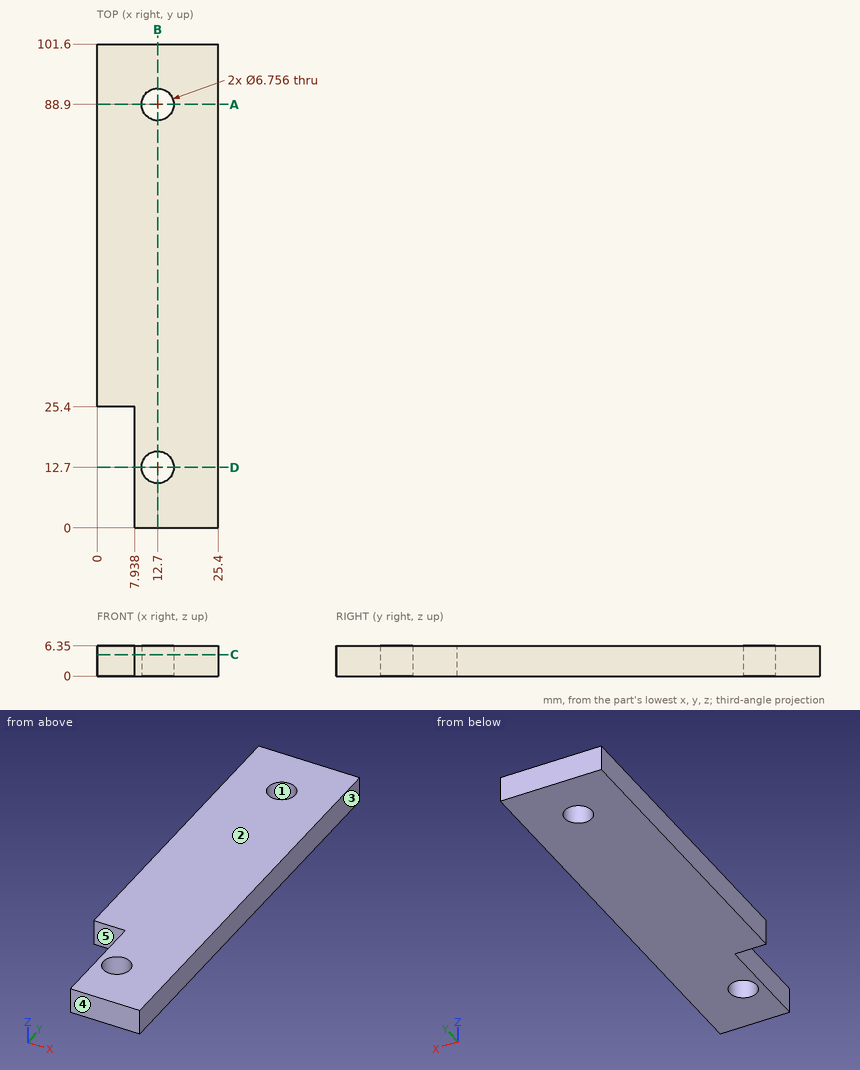
Design review of the part shown in the three views and the two pictorial views. Dimensions are in mm from the part's minimum x, y and z. A direction names the side the tool comes from. Round coordinates to 2 decimals unless told otherwise and drop trailing zeros. Loops run counter-clockwise (first coordinate to the right, second up) from the corner with the lowest first, then second, coordinate; pieces in that order, holes last.
Q1. To check wall thickness, follow line 1 along Y through (x, z) = (12.7, 3.75); line 2 along Y through (x, z) = (2.25, 3.5); line 3 along X through (y, z) = (7, 1). State the ranges of each line that lie inside material, in increasing order.
Result sheet:
line 1: y = 0 to 9.32, 16.08 to 85.52, 92.28 to 101.6
line 2: y = 25.4 to 101.6
line 3: x = 7.94 to 25.4
Q2. Add section D-D on y = 12.7. Write out the cut boundary in (x, z).
Result sheet:
outline: (7.94, 0) - (9.32, 0) - (9.32, 6.35) - (7.94, 6.35) - close; (16.08, 0) - (25.4, 0) - (25.4, 6.35) - (16.08, 6.35) - close
Q3. Mouldability with a two-part tool opening along X and no side actions: class the marked faces 1, 2 and 3 as +X half, -X half, draft (parallel to the pull), parting line (faces both ways), or undercut.
Result sheet:
face 1: undercut
face 2: draft
face 3: +X half
Q4. Add section C-C on z = 4.5. Write out the cut boundary in (x, y), plus the area to 3 significant figures.
Result sheet:
outline: (0, 25.4) - (7.94, 25.4) - (7.94, 0) - (25.4, 0) - (25.4, 101.6) - (0, 101.6) - close; hole circle Ø6.76 at (12.7, 12.7); hole circle Ø6.76 at (12.7, 88.9)
area: 2,310 mm2
Q5. Insertion check: pin 1 Ø3 at (x, z) = (3, 3) entering from -Y. The pin has a flat end and moves straight along its axis. Give the tip position at first contact, or say it passes through.
Result sheet:
pin 1: stops at y = 25.4
Q6. Machinability: for the marked faces 4 and 5, which of the approach directions +Z, -Z, +X, -X, +Y, -Y give a long, thin tool a straight path to every point of the face, cutting with its end or side? Answer none if there is none.
Result sheet:
face 4: +Z, -Z, +X, -X, -Y
face 5: +Z, -Z, -X, -Y
Q7. Add section B-B on x = 12.7. Write out the cut boundary in (y, z).
Result sheet:
outline: (0, 0) - (9.32, 0) - (9.32, 6.35) - (0, 6.35) - close; (16.08, 0) - (85.52, 0) - (85.52, 6.35) - (16.08, 6.35) - close; (92.28, 0) - (101.6, 0) - (101.6, 6.35) - (92.28, 6.35) - close
Q8. Add section A-A on y = 88.9. Write out the cut boundary in (x, z).
Result sheet:
outline: (0, 0) - (9.32, 0) - (9.32, 6.35) - (0, 6.35) - close; (16.08, 0) - (25.4, 0) - (25.4, 6.35) - (16.08, 6.35) - close
